Source: three-view drawing plus pictorial views. Frame: mm from the lowest corner of the part. Coordinates: 2 decimals unless noted, no trailing zeros. Write each loop counter-clockwise with the first axis right and the second up, starting at its lowest first coordinate (ties: lowest second). Pieces come first, ordered by that corner, then holes. Notation, with made-up numbers: (26, 14) -> (47, 14) arc R35 ccw to (47, 51) -> close; hole circle Ø7 at (-34, 23.5). An arc over 180 degrees is marked (long way). Write item = value, one per line.
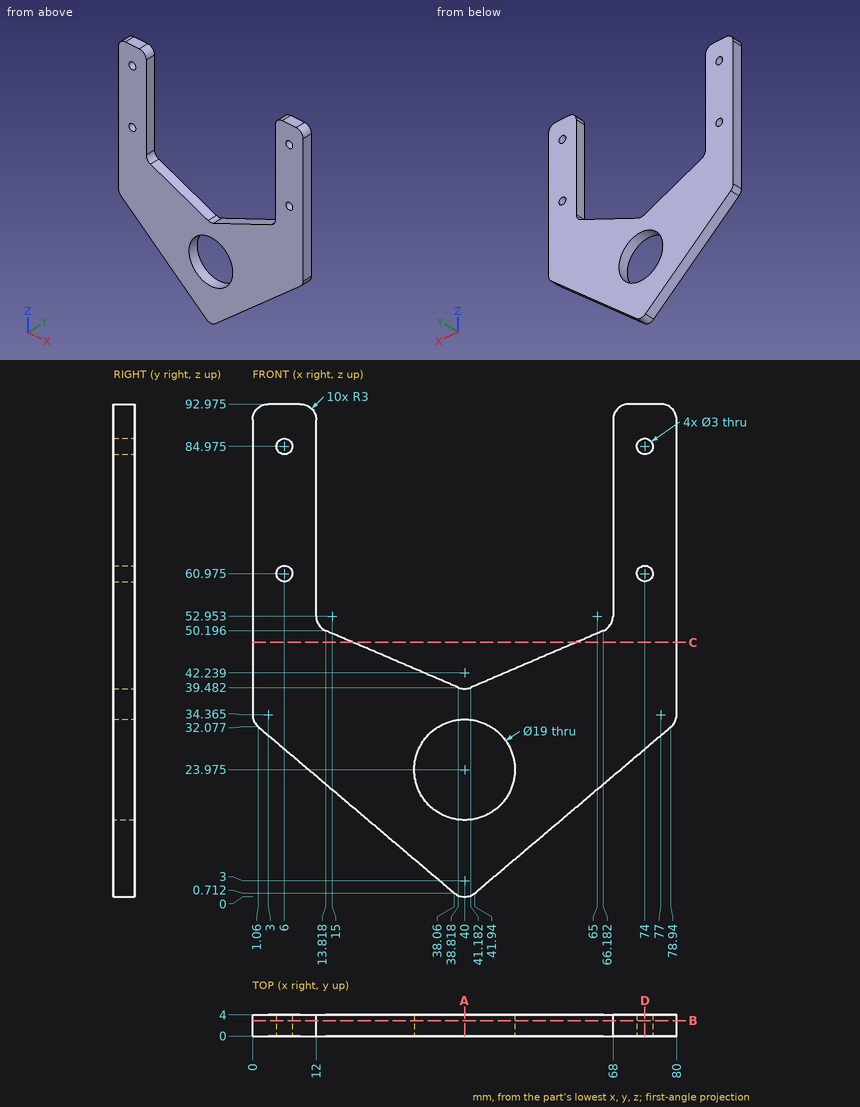
1) Cut plane C-C, the plane z = 48. Output: boundary loops of the cut face in (x, y).
Answer block:
outline = (0, 0) -> (18.94, 0) -> (18.94, 4) -> (0, 4) -> close; (61.06, 0) -> (80, 0) -> (80, 4) -> (61.06, 4) -> close
2) Cut plane A-A, the plane x = 40. Output: boundary loops of the cut face in (y, z) (1 decimal).
Answer block:
outline = (0, 0) -> (4, 0) -> (4, 14.5) -> (0, 14.5) -> close; (0, 33.5) -> (4, 33.5) -> (4, 39.2) -> (0, 39.2) -> close
3) Material intervals for probe 1 along X at (y, z) = (1.5, 85); probe 2 along Z at (x, y) = (74, 1.35) (1 decimal); probe 3 along X at (y, z) = (0.2, 84), sorted ascending. Write a range as [from, to].
Answer block:
probe_1 = [0, 4.5], [7.5, 12], [68, 72.5], [75.5, 80]
probe_2 = [27.9, 59.5], [62.5, 83.5], [86.5, 93]
probe_3 = [0, 4.86], [7.14, 12], [68, 72.86], [75.14, 80]
4) First-contact query: pin 1 Ø2.5 at (x, z) = (74, 84.98) entering from +Y. Flat tip, straight axial feed; report the tip coordinate or a pass-through.
Answer block:
pin_1 = through
5) Cut plane D-D, the plane x = 74. Output: boundary loops of the cut face in (y, z) (1 decimal), and give its area (3 significant figures).
Answer block:
outline = (0, 27.9) -> (4, 27.9) -> (4, 59.5) -> (0, 59.5) -> close; (0, 62.5) -> (4, 62.5) -> (4, 83.5) -> (0, 83.5) -> close; (0, 86.5) -> (4, 86.5) -> (4, 93) -> (0, 93) -> close
area = 236 mm2
6) Cut plane B-B, the plane y = 2.9. Output: boundary loops of the cut face in (x, z) (1 decimal).
Answer block:
outline = (0, 34.4) arc R3 ccw to (1.1, 32.1) -> (38.1, 0.7) arc R3 ccw to (41.9, 0.7) -> (78.9, 32.1) arc R3 ccw to (80, 34.4) -> (80, 90) arc R3 ccw to (77, 93) -> (71, 93) arc R3 ccw to (68, 90) -> (68, 53) arc R3 cw to (66.2, 50.2) -> (41.2, 39.5) arc R3 cw to (38.8, 39.5) -> (13.8, 50.2) arc R3 cw to (12, 53) -> (12, 90) arc R3 ccw to (9, 93) -> (3, 93) arc R3 ccw to (0, 90) -> close; hole circle Ø3 at (6, 61); hole circle Ø3 at (6, 85); hole circle Ø19 at (40, 24); hole circle Ø3 at (74, 61); hole circle Ø3 at (74, 85)
